from build123d import *

# Parameters (mm, degrees)
F1_DEPTH = 203.2
F2_W     = 44.45
F2_H     = 57.15
F3_DEPTH = 127.001
F4_R     = 12.69999


# Not quite as in the source:
# - a fillet or chamfer is up to 0.001 mm smaller than in the source, because OpenCascade refuses the exact size
# - a feature of the source that left no trace in its solid (it failed there, or was rolled back) is left out


with BuildPart() as f1:
    # F0 (on Top) → F1 (new body)
    with BuildSketch(Plane.XY):
        Polygon((-38.1, 0), (0, 0), (38.1, 0), (38.1, -44.45), (63.5, -44.45), (63.5, 50.8), (38.1, 50.8), (38.1, 6.35), (0, 6.35), (-38.1, 6.35), (-38.1, 50.8), (-63.5, 50.8), (-63.5, -44.45), (-38.1, -44.45), align=None)
    extrude(amount=F1_DEPTH)

    # F2 (on face) → F3 (cut, through all)
    with BuildSketch(Plane.YZ.offset(63.5)):
        with BuildLine():
            Line((-44.45, 115.316), (-44.45, 63.5))
            Line((-44.45, 63.5), (-1.5875, 63.5))
            ThreePointArc((-1.5875, 63.5), (-1.1225320151, 64.6225320151), (0, 65.0875))
            Line((0, 65.0875), (0, 113.7285))
            ThreePointArc((0, 113.7285), (-1.1225320151, 114.1934679849), (-1.5875, 115.316))
            Line((-1.5875, 115.316), (-44.45, 115.316))
        make_face()
        with BuildLine():
            ThreePointArc((0, 65.0875), (-1.1225320151, 64.6225320151), (-1.5875, 63.5))
            Line((-1.5875, 63.5), (0, 63.5))
            Line((0, 63.5), (0, 65.0875))
        make_face()
        with Locations((-22.225, 28.575)):
            Rectangle(F2_W, F2_H)
        Polygon((-44.45, 203.2), (-44.45, 184.15), (0, 195.7456521739), (0, 203.2), align=None)
        with BuildLine():
            Line((0, 115.316), (0, 113.7285))
            ThreePointArc((0, 113.7285), (1.1225320151, 114.1934679849), (1.5875, 115.316))
            ThreePointArc((1.5875, 115.316), (1.1225320151, 116.4385320151), (0, 116.9035))
            Line((0, 116.9035), (0, 115.316))
        make_face()
        with BuildLine():
            ThreePointArc((0, 116.9035), (-1.1225320151, 116.4385320151), (-1.5875, 115.316))
            Line((-1.5875, 115.316), (0, 115.316))
            Line((0, 115.316), (0, 116.9035))
        make_face()
        with BuildLine():
            Line((0, 115.316), (-1.5875, 115.316))
            ThreePointArc((-1.5875, 115.316), (-1.1225320151, 114.1934679849), (0, 113.7285))
            Line((0, 113.7285), (0, 115.316))
        make_face()
        with BuildLine():
            Line((0, 65.0875), (0, 63.5))
            Line((0, 63.5), (0, 61.9125))
            ThreePointArc((0, 61.9125), (1.1225320151, 62.3774679849), (1.5875, 63.5))
            ThreePointArc((1.5875, 63.5), (1.1225320151, 64.6225320151), (0, 65.0875))
        make_face()
        with BuildLine():
            Line((0, 63.5), (-1.5875, 63.5))
            ThreePointArc((-1.5875, 63.5), (-1.1225320151, 62.3774679849), (0, 61.9125))
            Line((0, 61.9125), (0, 63.5))
        make_face()
        Polygon((0, 203.2), (0, 195.7456521739), (28.575, 203.2), align=None)
        Polygon((-44.45, 184.15), (-44.45, 121.666), (0, 121.666), (0, 195.7456521739), align=None)
    extrude(amount=-F3_DEPTH, mode=Mode.SUBTRACT)

    # F4 (radius 12.7 in the source; OpenCascade refuses exactly that, so slightly less here)
    f4_edges = [f1.edges().sort_by_distance(p)[0] for p in [
        (38.1, -44.45, 118.491),
        (63.5, -44.45, 118.491),
        (-63.5, -44.45, 118.491),
        (-38.1, -44.45, 118.491),
        (-38.1, -44.45, 60.325),
        (-63.5, -44.45, 60.325),
        (38.1, -44.45, 60.325),
        (63.5, -44.45, 60.325),
    ]]
    fillet(f4_edges, radius=F4_R)


solid = f1.part
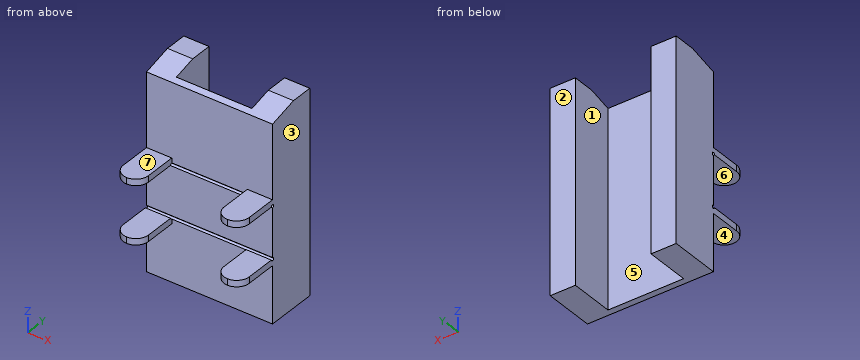
The model under review builds one solid part; all positions refer to its coordinate system, in mm. Face numbers are marked on the shaded views. A direction names the side the tool comes from. Give positions to 0.01 mm unless a question says otherwise; leave off trailing zeros. Order: outer loops, then holes, each group sorted by start corner. A loop starts at its lowest first (then second) coordinate and runs counter-clockwise, first axis right, second up. Notation, with made-up numbers: M 28,0 L 39,0 A10 cw 39,7 Z; hole C 71,55.25 d10. An arc over 180 degrees is marked long. Use one line per item in the form item = value. Start each with the question number.
Item 1: We need section B-B on z = 70. Give the boundary of the cut face in (x, y).
Item 2: We need section A-A on y = -29. Give the boundary of the cut face in (x, z), plus the area to 3 significant figures.
Item 3: The part is to be moulded in two halves that separate along X. For the marked faces 1, 2 and 3, say which applies: pulls with the +X half, pulls with the -X half, needs draft (parallel to the pull), parting line crosses it, or undercut.
Item 4: Insertion check: pin 1 Ø12 at (x, z) = (-5, 151) entering from -Y; pin 2 Ø7.5 at (x, y) = (51.5, -27.5) entering from -Z; pin 3 Ø7.5 at (x, y) = (-57, -32) entering from +Z. Each pin has a flat end and moves straight along its axis. Give the tip position at first contact, or say it passes through.
Item 5: For the marked faces 4, 5, 6 and 7, list the 3-axis set-ups (+Z, -Z, +X, -X, +Y, -Y) from which the entire face can be reached by the end or side of a thin tool; tool diameter is ignored.
Item 6: To check wall thickness, follow line 1 along X through (y, z) = (7, 92); line 2 along Z through (x, y) = (13, 1); line 3 along Z through (x, y) = (-46, -25). State the ranges of each line that lie inside material, in increasing order. Write a range as from..to.
Completed:
q1.outline = M -63.5,0 L 63.5,0 L 63.5,50.8 L 38.1,50.8 L 38.1,6.35 L -38.1,6.35 L -38.1,50.8 L -63.5,50.8 Z
q2.outline = M -63.5,57.15 L -38.1,57.15 L -38.1,63.5 L -63.5,63.5 Z; M -63.5,115.32 L -38.1,115.32 L -38.1,121.67 L -63.5,121.67 Z; M 38.1,57.15 L 63.5,57.15 L 63.5,63.5 L 38.1,63.5 Z; M 38.1,115.32 L 63.5,115.32 L 63.5,121.67 L 38.1,121.67 Z
q2.area = 645 mm²
q3.face_1 = undercut
q3.face_2 = needs draft
q3.face_3 = pulls with the +X half
q4.pin_1 = 0
q4.pin_2 = 57.15
q4.pin_3 = 121.67
q5.face_4 = -Z, +X, -X, -Y
q5.face_5 = +Z, -Z, +Y
q5.face_6 = +X, -X, -Y
q5.face_7 = +Z, +X, -X, -Y
q6.line_1 = -63.5..-38.1, 38.1..63.5
q6.line_2 = 0..62.27, 64.73..114.08, 116.55..196.01
q6.line_3 = 57.15..63.5, 115.32..121.67
